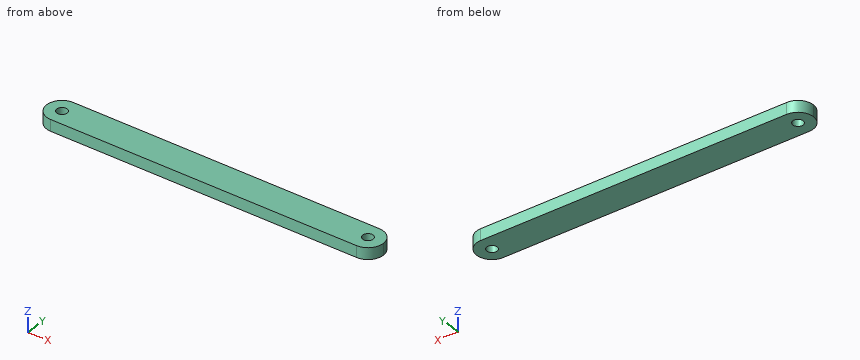
```python
from build123d import *

# Parameters (mm, degrees)
SKETCH_1_R      = 1.354010502
EXTRUDE_1_DEPTH = 3


with BuildPart() as part:
    # 草图1 → 凸台-拉伸1 (new body)
    with BuildSketch(Plane(origin=(0, 0, 0), x_dir=(-1, 0, 0), z_dir=(0, 0, -1))):
        with BuildLine():
            Line((-55.860221974, 0), (24.13832066, 0))
            ThreePointArc((24.13832066, 0), (26.966394209, 1.171219344), (28.138320535, 3.999))
            ThreePointArc((28.138320535, 3.999), (26.96674766, 6.827427125), (24.138320535, 7.999))
            Line((24.138320535, 7.999), (-55.860222099, 7.999))
            ThreePointArc((-55.860222099, 7.999), (-58.688295648, 6.827780656), (-59.860221974, 4))
            ThreePointArc((-59.860221974, 4), (-58.688649099, 1.171572875), (-55.860221974, 0))
        make_face()
        with Locations((24.138809001, 3.998511534)):
            Circle(SKETCH_1_R, mode=Mode.SUBTRACT)
        with Locations((-55.859733508, 3.999511534)):
            Circle(SKETCH_1_R, mode=Mode.SUBTRACT)
    extrude(amount=-EXTRUDE_1_DEPTH)


solid = part.part
```
Model file for the job. Use its own axes, mm. Coordinates: 2 decimals unless noted, no trailing zeros. Write each loop counter-clockwise with the first axis right and the second up, starting at its lowest first coordinate (ties: lowest second). Pieces come first, ordered by that corner, then holes. Notation, with made-up numbers: (41.25, 77) - (59.25, 77) arc R19 cw to (59.25, 93) - close; hole circle Ø2 at (-28.75, 28). An arc over 180 degrees is marked (long way). One line per item, written item: value. Start each with the question number.
1. Probe line 1 (X direction, y = 4, z = 0.5); line 2 (X direction, y = 4.75, z = 1); line 3 (X direction, y = 0.5, z = 0.75). List the from-to ranges inside material, lowest first. Write a range as from..to.
2. Slice it at A-A (z = 1.25). Write the cut outline in (x, y), plus the area to 3 significant figures.
3. Flat gauge pin, fed straight in: pin 1 (1.5 mm diameter, centred on y = 3, z = 2, fed in from -X). Where does the tip first touch, or does it go through?
Answers below:
1. line 1: x = -28.14..-25.49, -22.78..54.51, 57.21..59.86
1. line 2: x = -28.07..-25.27, -23.01..54.73, 56.99..59.79
1. line 3: x = -26.07..57.8
2. outline: (-28.14, 4) arc R4 ccw to (-24.14, 0) - (55.86, 0) arc R4 ccw to (59.86, 4) arc R4 ccw to (55.86, 8) - (-24.14, 8) arc R4 ccw to start; hole circle Ø2.71 at (-24.14, 4); hole circle Ø2.71 at (55.86, 4)
2. area: 679 mm^2
3. pin 1: stops at x = -28.13
